For this review, take the finished solid that the model builds, in its own axes (mm). Face numbers are marked on the shaded views. A direction names the side the tool comes from. Give positions to 0.01 mm unless a question says otherwise; leave off trailing zeros. Write each loop counter-clockwise with the first axis right and the second up, starting at its lowest first coordinate (ties: lowest second). Pieces come first, ordered by that corner, then holes. Notation, with made-up numbers: M -29,79.5 L 7,79.5 A21 cw 7,105.5 Z; hole C -16,4.25 d2. An arc over 180 degrees is marked long. Answer as a JSON object with one key per item and string values. Group by question number.
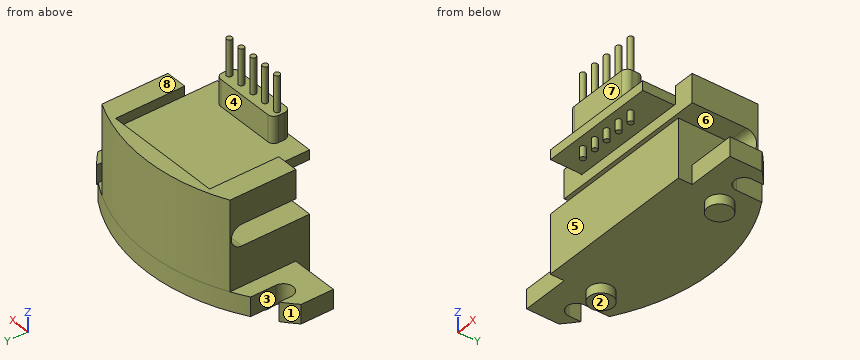
```python
from build123d import *

# Parameters (mm, degrees)
BOSS_EXTRU_1_DEPTH           = 1.6
BOSS_EXTRU_2_DEPTH           = 7.48
ESQUISSE3_W                  = 10
ESQUISSE3_H                  = 5.8
ENL_V_MAT_EXTRU_2_DEPTH      = 1.5
ENL_V_MAT_EXTRU_3_DEPTH      = 18.6
ESQUISSE5_R                  = 1
BOSS_EXTRU_3_DEPTH           = 0.8
ESQUISSE8_W                  = 0.23
ESQUISSE8_H                  = 6.92
R_P_TITION_LIN_AIRE1_COUNT   = 3
R_P_TITION_LIN_AIRE1_PITCH   = 1.27
R_P_TITION_LIN_AIRE1_2_COUNT = 3
R_P_TITION_LIN_AIRE1_2_PITCH = 1.27
BOSS_EXTRU_4_DEPTH           = 0.8
ESQUISSE11_W                 = 13.6
ESQUISSE11_H                 = 1.17
BOSS_EXTRU_5_DEPTH           = 4.9
BOSS_EXTRU_6_DEPTH           = 2.22


with BuildPart() as part:
    # Esquisse1 → Boss.-Extru.1 (new body)
    with BuildSketch(Plane.XY):
        with BuildLine():
            Line((-10.8, 0.018003418), (-10.8, -2.69))
            Line((-10.8, -2.69), (10.8, -2.69))
            Line((10.8, -2.69), (10.8, 0.018003418))
            ThreePointArc((10.8, 0.018003418), (10.261507275, 0.516861385), (9.7, 0.989665008))
            Line((9.7, 0.989665008), (9.7, 0))
            ThreePointArc((9.7, 0), (8.9, -0.8), (8.1, 0))
            Line((8.1, 0), (8.1, 2.115142829))
            ThreePointArc((8.1, 2.115142829), (0, 4.4), (-8.1, 2.115142829))
            Line((-8.1, 2.115142829), (-8.1, 0))
            ThreePointArc((-8.1, 0), (-8.9, -0.8), (-9.7, 0))
            Line((-9.7, 0), (-9.7, 0.989665008))
            ThreePointArc((-9.7, 0.989665008), (-10.261507275, 0.516861385), (-10.8, 0.018003418))
        make_face()
    extrude(amount=BOSS_EXTRU_1_DEPTH)

    # Esquisse2 → Boss.-Extru.2 (add)
    with BuildSketch(Plane.XY.offset(1.6)):
        with BuildLine():
            Line((-6.8, 2.828747252), (-6.8, -2.69))
            Line((-6.8, -2.69), (6.8, -2.69))
            Line((6.8, -2.69), (6.8, 2.828747252))
            ThreePointArc((6.8, 2.828747252), (0, 4.4), (-6.8, 2.828747252))
        make_face()
    extrude(amount=BOSS_EXTRU_2_DEPTH)

    # Esquisse3 → Enl_v. mat.-Extru.2 (cut)
    with BuildSketch(Plane.XY.offset(9.08)):
        with Locations((0, 0.21)):
            Rectangle(ESQUISSE3_W, ESQUISSE3_H)
    extrude(amount=-ENL_V_MAT_EXTRU_2_DEPTH, mode=Mode.SUBTRACT)

    # Esquisse4 → Enl_v. mat.-Extru.3 (cut, through all)
    with BuildSketch(Plane.ZY.offset(6.8)):
        with BuildLine():
            Line((4.9, -2.69), (4.9, 1.828747252))
            ThreePointArc((4.9, 1.828747252), (5.79, 2.718747252), (6.68, 1.828747252))
            Line((6.68, 1.828747252), (6.68, -2.69))
            ThreePointArc((6.68, -2.69), (5.79, -3.58), (4.9, -2.69))
        make_face()
    extrude(amount=-ENL_V_MAT_EXTRU_3_DEPTH, mode=Mode.SUBTRACT)

    # Esquisse5 → Boss.-Extru.3 (add)
    with BuildSketch(Plane(origin=(0, 0, 0), x_dir=(-1, 0, 0), z_dir=(0, 0, -1))):
        with Locations((6.3, 0)):
            Circle(ESQUISSE5_R)
        with Locations((-6.3, 0)):
            Circle(ESQUISSE5_R)
    extrude(amount=BOSS_EXTRU_3_DEPTH)



with BuildPart() as body_2:
    # Esquisse8 → R_volution1 (revolve)
    with BuildSketch(Plane(origin=(0, -4.49, 0), x_dir=(1, 0, 0), z_dir=(0, 1, 0))):
        with Locations((0.115, -10.14)):
            Rectangle(ESQUISSE8_W, ESQUISSE8_H)
    revolve(axis=Axis((0, -4.49, 7.58), (0, 0, 1)))


with BuildPart() as r_p_tition_lin_aire1_1:
    # R_p_tition lin_aire1: pattern copy
    add(body_2.part.moved(Location(Vector(1, 0, 0) * (1 * R_P_TITION_LIN_AIRE1_PITCH))))


with BuildPart() as r_p_tition_lin_aire1_2:
    # R_p_tition lin_aire1: pattern copy
    add(body_2.part.moved(Location(Vector(1, 0, 0) * (2 * R_P_TITION_LIN_AIRE1_PITCH))))


with BuildPart() as r_p_tition_lin_aire1_2_1:
    # R_p_tition lin_aire1 2: pattern copy
    add(body_2.part.moved(Location(Vector(-1, 0, 0) * (1 * R_P_TITION_LIN_AIRE1_2_PITCH))))


with BuildPart() as r_p_tition_lin_aire1_2_2:
    # R_p_tition lin_aire1 2: pattern copy
    add(body_2.part.moved(Location(Vector(-1, 0, 0) * (2 * R_P_TITION_LIN_AIRE1_2_PITCH))))


with BuildPart() as r_p_tition_lin_aire1_2_3:
    # R_p_tition lin_aire1 2: pattern copy
    add(r_p_tition_lin_aire1_1.part.moved(Location(Vector(-1, 0, 0) * (1 * R_P_TITION_LIN_AIRE1_2_PITCH))))


with BuildPart() as r_p_tition_lin_aire1_2_4:
    # R_p_tition lin_aire1 2: pattern copy
    add(r_p_tition_lin_aire1_1.part.moved(Location(Vector(-1, 0, 0) * (2 * R_P_TITION_LIN_AIRE1_2_PITCH))))


with BuildPart() as r_p_tition_lin_aire1_2_5:
    # R_p_tition lin_aire1 2: pattern copy
    add(r_p_tition_lin_aire1_2.part.moved(Location(Vector(-1, 0, 0) * (1 * R_P_TITION_LIN_AIRE1_2_PITCH))))


with BuildPart() as r_p_tition_lin_aire1_2_6:
    # R_p_tition lin_aire1 2: pattern copy
    add(r_p_tition_lin_aire1_2.part.moved(Location(Vector(-1, 0, 0) * (2 * R_P_TITION_LIN_AIRE1_2_PITCH))))


with BuildPart() as part_1:
    add(part.part)

    add(body_2.part)  # Boss.-Extru.4 merges body 2

    add(r_p_tition_lin_aire1_1.part)  # Boss.-Extru.4 merges R_p_tition lin_aire1_1

    add(r_p_tition_lin_aire1_2.part)  # Boss.-Extru.4 merges R_p_tition lin_aire1_2

    add(r_p_tition_lin_aire1_2_1.part)  # Boss.-Extru.4 merges R_p_tition lin_aire1 2_1

    add(r_p_tition_lin_aire1_2_2.part)  # Boss.-Extru.4 merges R_p_tition lin_aire1 2_2

    add(r_p_tition_lin_aire1_2_3.part)  # Boss.-Extru.4 merges R_p_tition lin_aire1 2_3

    add(r_p_tition_lin_aire1_2_4.part)  # Boss.-Extru.4 merges R_p_tition lin_aire1 2_4

    add(r_p_tition_lin_aire1_2_5.part)  # Boss.-Extru.4 merges R_p_tition lin_aire1 2_5

    add(r_p_tition_lin_aire1_2_6.part)  # Boss.-Extru.4 merges R_p_tition lin_aire1 2_6
    # Esquisse10 → Boss.-Extru.4 (add)
    with BuildSketch(Plane.XY.offset(7.58)):
        Polygon((-4.9, -2.59), (-4.9, -5.34), (4.9, -5.34), (4.9, -2.59), (4.9, 3.01), (-4.9, 3.01), align=None)
    extrude(amount=BOSS_EXTRU_4_DEPTH)

    # Esquisse11 → Boss.-Extru.5 (add)
    with BuildSketch(Plane(origin=(0, 0, 0), x_dir=(-1, 0, 0), z_dir=(0, 0, -1))):
        with Locations((0, -3.275)):
            Rectangle(ESQUISSE11_W, ESQUISSE11_H)
    extrude(amount=-BOSS_EXTRU_5_DEPTH)

    # Esquisse12 → Boss.-Extru.6 (add)
    with BuildSketch(Plane.XY.offset(8.38)):
        with BuildLine():
            Line((2.5, -5.24), (-2.5, -5.24))
            ThreePointArc((-2.5, -5.24), (-2.853553391, -5.093553391), (-3, -4.74))
            Line((-3, -4.74), (-3, -4.24))
            ThreePointArc((-3, -4.24), (-2.853553391, -3.886446609), (-2.5, -3.74))
            Line((-2.5, -3.74), (2.5, -3.74))
            ThreePointArc((2.5, -3.74), (2.853553391, -3.886446609), (3, -4.24))
            Line((3, -4.24), (3, -4.74))
            ThreePointArc((3, -4.74), (2.853553391, -5.093553391), (2.5, -5.24))
        make_face()
    extrude(amount=BOSS_EXTRU_6_DEPTH)


solid = part_1.part
```
Item 1: Insertion check: P1, Ø1.3, axis at x = 9, z = 1, coming from the -Y side; P2, Ø4, axis at x = -2.5, y = -2, coming from the +Z side; P3, Ø1.3, axis at x = 1.5, y = -4, coming from the -Z side. Each pin has a flat end and moves straight along its axis. Give the tip position at first contact, or say it passes through.
Item 2: Consider section D-D (y = -0.25). State how many separate pieces and enclosed holes the cut face has, plus the area to 3 significant figures.
Item 3: Draft analysis for pull direction X (two halves, no side actions). For the marked faces 1, 2 and 3, state which applies: released by +X, released by -X, zero draft, split by the parting line, or undercut.
Item 4: To check wall thickness, follow probe 1 along Z at (x, y) = (2.25, 0); probe 2 along Z at (x, y) = (6, 0.75); probe 3 along X at (y, z) = (-3, 0.5). State the ranges of each line that lie inside material, in increasing order.
Item 5: Consider section C-C (z = 1.25). Give the boundary of the cut face in (x, y), plus the area to 3 significant figures.
Item 6: Consider section A-A (y = -1.5). Give the boundary of the cut face in (x, z).
Item 7: Consider section B-B (x = 0). Give the boundary of the cut face in (y, z), plus the area to 3 significant figures.
Item 8: Machinability: for the marked faces 4, 5, 6, 7 and 8, which of the approach directions +Z, -Z, +X, -X, +Y, -Y give a long, thin tool a straight path to every point of the face, cutting with its end or side? Answer none if there is none.
Result set:
{
 "1": {"P1": "stops at y = -2.69", "P2": "stops at z = 10.6", "P3": "stops at z = 0"},
 "2": {"separate pieces": "4", "enclosed holes": "0", "area": "103 mm^2"},
 "3": {"face 1": "released by -X", "face 2": "zero draft", "face 3": "undercut"},
 "4": {"probe 1": "z = 0 to 4.9, 6.68 to 8.38", "probe 2": "z = -0.8 to 4.9, 6.68 to 9.08", "probe 3": "x = -6.8 to 6.8"},
 "5": {"outline": "M -10.8,-2.69 L -6.8,-2.69 L -6.8,-3.86 L 6.8,-3.86 L 6.8,-2.69 L 10.8,-2.69 L 10.8,0.02 A15.5 ccw 9.7,0.99 L 9.7,0 A0.8 cw 8.1,0 L 8.1,2.12 A15.5 ccw -8.1,2.12 L -8.1,0 A0.8 cw -9.7,0 L -9.7,0.99 A15.5 ccw -10.8,0.02 Z", "area": "132 mm^2"},
 "6": {"outline": "M -10.8,0 L 10.8,0 L 10.8,1.6 L 6.8,1.6 L 6.8,4.9 L -6.8,4.9 L -6.8,1.6 L -10.8,1.6 Z; M -6.8,6.68 L 6.8,6.68 L 6.8,9.08 L 5,9.08 L 5,7.58 L 4.9,7.58 L 4.9,8.38 L -4.9,8.38 L -4.9,7.58 L -5,7.58 L -5,9.08 L -6.8,9.08 Z"},
 "7": {"outline": "M -5.34,7.58 L -4.72,7.58 L -4.72,6.68 L -4.26,6.68 L -4.26,7.58 L -2.69,7.58 L -2.69,6.68 L 1.83,6.68 A0.89 cw 1.83,4.9 L -3.86,4.9 L -3.86,0 L 4.4,0 L 4.4,9.08 L 3.11,9.08 L 3.11,7.58 L 3.01,7.58 L 3.01,8.38 L -3.74,8.38 L -3.74,10.6 L -4.26,10.6 L -4.26,13.6 L -4.72,13.6 L -4.72,10.6 L -5.24,10.6 L -5.24,8.38 L -5.34,8.38 Z", "area": "63.9 mm^2"},
 "8": {"face 4": "+Z, +X, -X", "face 5": "-Z, +X, -X, -Y", "face 6": "+X, -X, -Y", "face 7": "+Z, +X, -X, -Y", "face 8": "+Z, +X, -X, +Y"}
}
